Work out the finished part from the listing and answer in its coordinate system (mm). A direction names the side the tool comes from. Round coordinates to 2 decimals unless told otherwise and drop trailing zeros. Order: outer loops, then holes, each group sorted by start corner. A loop starts at its lowest first (then second) coordinate and runs counter-clockwise, first axis right, second up. Notation, with made-up numbers: M 77,22 L 121,22 A19 ccw 121,48 Z; hole C -2.75,83 d2. An arc over 180 degrees is marked long. Return JSON: item names as keys, results as strings.
from build123d import *

# Parameters (mm, degrees)
SKETCH_1_R          = 1.6
SKETCH_1_W          = 25.85
SKETCH_1_H          = 47
EXTRUDE_1_DEPTH     = 4
SKETCH_2_W          = 8
SKETCH_2_H          = 6
SKETCH_2_R          = 1.6
EXTRUDE_2_DEPTH     = 17
FILLET_1_R          = 2
SKETCH_3_W          = 132.85
SKETCH_3_H          = 6
EXTRUDE_3_DEPTH     = 29
SKETCH_4_W          = 10
SKETCH_4_H          = 22
CUT_EXTRUDE_1_DEPTH = 7
SKETCH_5_R          = 1.6
CUT_EXTRUDE_2_DEPTH = 34
SKETCH_6_R          = 1.6
CUT_EXTRUDE_3_DEPTH = 7


with BuildPart() as part:
    # Эскиз1 → Бобышка-Вытянуть1 (new body)
    with BuildSketch(Plane(origin=(0, 0, 0), x_dir=(1, 0, 0), z_dir=(0, 1, 0))):
        Polygon((66, 24), (66, -56), (-66.85, -56), (-66.85, 3), (-59.15, 3), (-34.85, 3), (-27.15, 3), (-27.15, -50), (27.704212942, -50), (40.133263836, 24), (60, 24), align=None)
        with Locations((63, 21)):
            Circle(SKETCH_1_R, mode=Mode.SUBTRACT)
        with Locations((-63, 0)):
            Circle(SKETCH_1_R, mode=Mode.SUBTRACT)
        with Locations((-31, 0)):
            Circle(SKETCH_1_R, mode=Mode.SUBTRACT)
        with Locations((43, 21)):
            Circle(SKETCH_1_R, mode=Mode.SUBTRACT)
        with Locations((-46.075, -26.5)):
            Rectangle(SKETCH_1_W, SKETCH_1_H, mode=Mode.SUBTRACT)
        Polygon((60, 18), (60, -50), (34.802263374, -50), (46.223553385, 18), align=None, mode=Mode.SUBTRACT)
    extrude(amount=EXTRUDE_1_DEPTH)

    # Эскиз2 → Бобышка-Вытянуть2 (add)
    with BuildSketch(Plane.XZ):
        with Locations((-62.85, 0)):
            Rectangle(SKETCH_2_W, SKETCH_2_H)
        with Locations((-63, 0)):
            Circle(SKETCH_2_R, mode=Mode.SUBTRACT)
        Polygon((66, -20), (66, -24), (60, -24), (60, -18), (64, -18), align=None)
        with Locations((63, -21)):
            Circle(SKETCH_2_R, mode=Mode.SUBTRACT)
        with Locations((-31.15, 0)):
            Rectangle(SKETCH_2_W, SKETCH_2_H)
        with Locations((-31, 0)):
            Circle(SKETCH_2_R, mode=Mode.SUBTRACT)
        Polygon((46.223553385, -18), (46.223553385, -24), (40.133263836, -24), (39.097062378, -17.830670696), (46.195112811, -17.830670696), align=None)
        with Locations((43, -21)):
            Circle(SKETCH_2_R, mode=Mode.SUBTRACT)
    extrude(amount=EXTRUDE_2_DEPTH)

    # Скругление1
    fillet_1_edges = [part.edges().sort_by_distance(p)[0] for p in [
        (-27.15, -6.5, -3),
        (40.133263836, -6.5, -24),
    ]]
    fillet(fillet_1_edges, radius=FILLET_1_R)

    # Эскиз3 → Бобышка-Вытянуть3 (add)
    with BuildSketch(Plane.XZ):
        with Locations((-0.425, 53)):
            Rectangle(SKETCH_3_W, SKETCH_3_H)
    extrude(amount=EXTRUDE_3_DEPTH)

    # Эскиз4 → Вырез-Вытянуть1 (cut, through all)
    with BuildSketch(Plane(origin=(0, 0, 50), x_dir=(-1, 0, 0), z_dir=(0, 0, -1))):
        with Locations((20.095331259, -13)):
            Rectangle(SKETCH_4_W, SKETCH_4_H)
        with Locations((2.321498445, -13)):
            Rectangle(SKETCH_4_W, SKETCH_4_H)
        with Locations((-15.45233437, -13)):
            Rectangle(SKETCH_4_W, SKETCH_4_H)
        with Locations((-33.226167185, -13)):
            Rectangle(SKETCH_4_W, SKETCH_4_H)
        with Locations((-51, -13)):
            Rectangle(SKETCH_4_W, SKETCH_4_H)
        with Locations((37.869164074, -13)):
            Rectangle(SKETCH_4_W, SKETCH_4_H)
        with Locations((55.642996889, -13)):
            Rectangle(SKETCH_4_W, SKETCH_4_H)
    extrude(amount=-CUT_EXTRUDE_1_DEPTH, mode=Mode.SUBTRACT)

    # Эскиз5 → Вырез-Вытянуть2 (cut, through all)
    with BuildSketch(Plane(origin=(0, 4, 0), x_dir=(1, 0, 0), z_dir=(0, 1, 0))):
        with Locations((-62.85, -53)):
            Circle(SKETCH_5_R)
        with Locations((-28.85, -53)):
            Circle(SKETCH_5_R)
        with Locations((63, -53)):
            Circle(SKETCH_5_R)
        with Locations((25, -53)):
            Circle(SKETCH_5_R)
    extrude(amount=-CUT_EXTRUDE_2_DEPTH, mode=Mode.SUBTRACT)

    # Эскиз6 → Вырез-Вытянуть3 (cut, through all)
    with BuildSketch(Plane(origin=(0, 0, 50), x_dir=(-1, 0, 0), z_dir=(0, 0, -1))):
        with Locations((46.075, -14)):
            Circle(SKETCH_6_R)
        with Locations((-59, -14)):
            Circle(SKETCH_6_R)
    extrude(amount=-CUT_EXTRUDE_3_DEPTH, mode=Mode.SUBTRACT)


solid = part.part
Item 1: Find section A-A (x = -1.5). Determine the outline of the cut face in (y, z).
Output:
{"outline": "M -29,50 L -24,50 L -24,56 L -29,56 Z; M -2,50 L 4,50 L 4,56 L -2,56 Z"}
Item 2: Find section C-C (z = 41.5). Determine the outline of the cut face in (x, y), plus the area to 3 significant figures.
Output:
{"outline": "M -66.85,0 L -59,0 L -59,4 L -66.85,4 Z; M -33.15,0 L -27.15,0 L -27.15,4 L -33.15,4 Z; M 29.13,0 L 36.23,0 L 36.23,4 L 29.13,4 Z; M 60,0 L 66,0 L 66,4 L 60,4 Z", "area": "108 mm^2"}
Item 3: The mould has two halves that part along Y. Classify faces 1 (the flat face through (-52, 1, -3)), 2 (the flat face through (61.7, -17, -22.3)), 3 (the flat face through (-20, -24, 53)): pulls with the +Y half, pulls with the -Y half, needs draft (parallel to the pull), parting line crosses it, or undercut.
Output:
{"face 1": "needs draft", "face 2": "pulls with the -Y half", "face 3": "undercut"}
Item 4: Find section B-B (y = -3.5). State how many separate pieces and enclosed holes the cut face has, plus the area to 3 significant figures.
Output:
{"separate pieces": "12", "enclosed holes": "8", "area": "482 mm^2"}
Item 5: Which of the six approach directions +Z, -Z, +X, -X, +Y, -Y give full straight-line access (tool end or side, diameter ignored) to faces 4 (the flat face through (-33.15, 2, 27)), 5 (the flat face through (62, -8, -18)), 6 (the flat face through (-47, 1, 3)), 7 (the flat face through (20.452, -13, 53)), 8 (the flat face through (-1, -1, 56))?
Output:
{"face 4": "+Y, -Y", "face 5": "+X, -Y", "face 6": "-Y", "face 7": "+Z, -Z", "face 8": "+Z, +X, -X, +Y, -Y"}
Item 6: Each of these flat-tipped pins is pushed along its axis until it touches: pin 1 (12 mm diameter, centred on x = -4, y = -8.5, fed in from +Z); pin 2 (12 mm diameter, centred on x = -41, z = -3, fed in from -Y); pin 3 (10 mm diameter, centred on x = 9.5, y = -5.5, fed in from -Z); pin 4 (2 mm diameter, centred on x = -24.5, z = 36, fed in from -Y). Where does it stop, or does it pass through?
Output:
{"pin 1": "stops at z = 56", "pin 2": "stops at y = -17", "pin 3": "stops at z = 50", "pin 4": "passes through"}
Item 7: Consider line 1 along Z through (x, y) = (-63, -7); line 2 along Z through (x, y) = (43, -10.5); line 3 along Z through (x, y) = (63, -10.5). Determine where each line is inside the solid, lowest interval first. Write a range as [from, to].
Output:
{"line 1": "z = [-3, -1.6], [1.6, 3], [50, 51.41], [54.59, 56]", "line 2": "z = [-24, -22.6], [-19.4, -17.83], [50, 56]", "line 3": "z = [-24, -22.6], [-19.4, -18], [50, 51.4], [54.6, 56]"}
